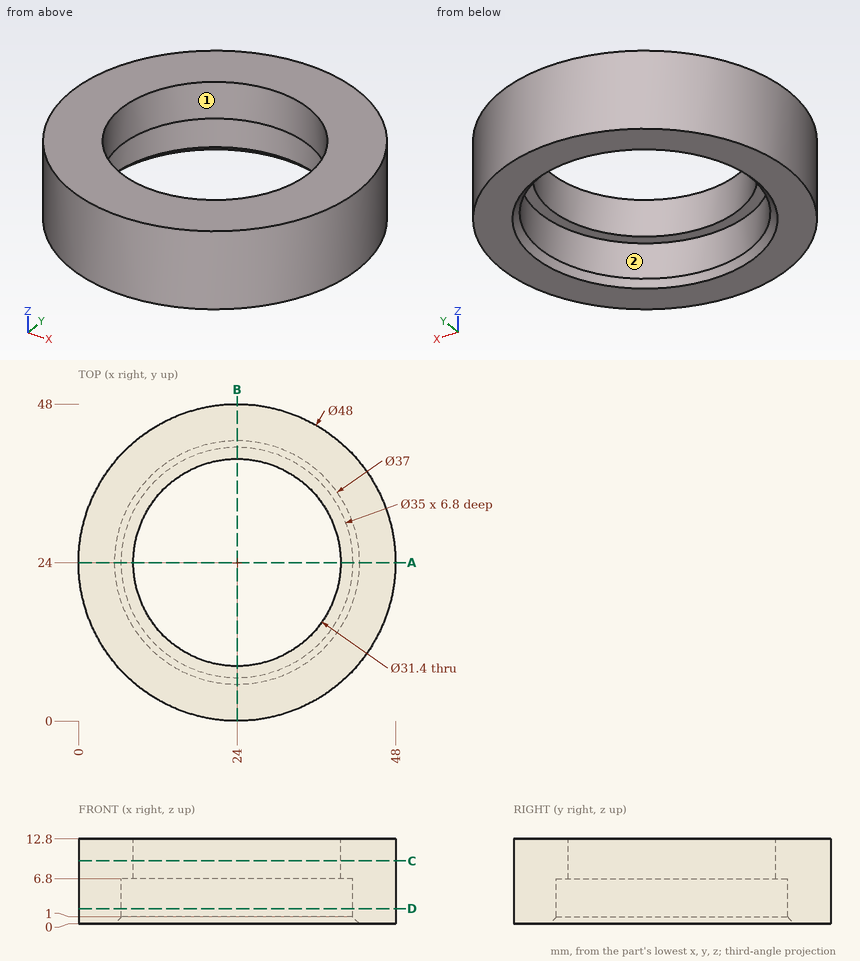
Verification items for this drawing (mm, ordinates from the low corner). A direction names the side the tool comes from. Give positions to 0.01 mm unless a question says otherwise; leave off trailing zeros. Order: outer loops, then holes, each group sorted by start corner. A loop starts at its lowest first (then second) coordinate and runs counter-clockwise, first axis right, second up. Notation, with made-up numbers: M -18,-11 L 11,-11 A34 cw 11,24 Z; hole C -33,84 d7. An arc over 180 degrees is marked long. Use a Markdown table: item, result.
Item 1: Depth check by flat-ended pin: P1, Ø8, axis at x = 8, y = 22.5, coming from the -Z side; P2, Ø1, axis at y = 31.5, z = 1.5, coming from the -X side; P3, Ø1, axis at x = 35, z = 9.5, coming from the -Y side; P4, Ø3, axis at x = 21.5, z = 4.5, coming from the +Y side. Enter the tip coordinate at first touch or a pass-through.
Answers follow:
| item | result |
|---|---|
| P1 | stops at z = 0 |
| P2 | stops at x = 1.04 |
| P3 | stops at y = 2.42 |
| P4 | stops at y = 47.98 |
Item 2: Tool access check on the marked faces 1 and 2. Record the directions out of +Z, -Z, +X, -X, +Y, -Y that give a thin tool (end or side, any length) a straight path to the whole face; none if there is none.
Answers follow:
| item | result |
|---|---|
| face 1 | +Z, -Z |
| face 2 | -Z |
Item 3: Section check C-C (z = 9.5). Record the cut outline in (x, y), and give its area (3 significant figures).
Answers follow:
| item | result |
|---|---|
| outline | C 24,24 d48; hole C 24,24 d31.4 |
| area | 1,040 mm2 |
Item 4: Section check A-A (y = 24). Record the cut outline in (x, z), and give its area (3 significant figures).
Answers follow:
| item | result |
|---|---|
| outline | M 0,0 L 5.5,0 L 6.5,1 L 6.5,6.8 L 8.3,6.8 L 8.3,12.8 L 0,12.8 Z; M 39.7,6.8 L 41.5,6.8 L 41.5,1 L 42.5,0 L 48,0 L 48,12.8 L 39.7,12.8 Z |
| area | 187 mm2 |
Item 5: Material ranges on line 1 along X through (y, z) = (24, 9.5); line 2 along Y through (x, z) = (11.5, 4.5), recorded low to high.
Answers follow:
| item | result |
|---|---|
| line 1 | x = 0 to 8.3, 39.7 to 48 |
| line 2 | y = 3.51 to 11.75, 36.25 to 44.49 |
Item 6: Section check D-D (z = 2.25). Record the cut outline in (x, y), and give its area (3 significant figures).
Answers follow:
| item | result |
|---|---|
| outline | C 24,24 d48; hole C 24,24 d35 |
| area | 847 mm2 |
